Can you work these out from the model? Positions are in its coordinate system, mm. Give positions to 0.01 mm unless a question says otherwise; leave off trailing zeros. Loops run counter-clockwise (first coordinate to the right, second up) from the corner with the lowest first, then second, coordinate; pieces in that order, holes last. Notation, with made-up numbers: (72.25, 72) -> (91.25, 72) arc R24 ccw to (91.25, 102) -> close; hole circle Ø1 at (65, -29). An arc over 180 degrees is marked (long way). Return JSON: item names as keys, results as strings. Group by question number.
Q1. Suppose I cut it at B-B, the plane x = 0. Please give me the cut outline in (y, z), and give its area (3 significant figures).
Q2. Suppose I cut it at C-C, the plane z = 1.3. Please give me the cut outline in (x, y).
Q3. Suppose I cut it at A-A, the plane y = 0. Please give me the cut outline in (x, z), and give its area (3 significant figures).
Q4. I need wall thicknesses on line 1 along X through (y, z) = (2, 0.7); line 2 along X through (y, z) = (25.5, 2.9); line 3 along Y through (x, z) = (29, 0.85). Which ranges of each line are inside material? Lowest first, please. Write a range as [from, to].
Q5. Thinking about a two-plate mould opening in Y: for faces 1 (the flat face through (18, 1, 3)), 2 (the cylindrical face through (24, 0, 1)), 3 (the cylindrical face through (-15.584, 20.234, 1.479)), 4 (the cylindrical face through (-64.49, 59.14, 1.48)), which applies, pulls with the +Y half, pulls with the -Y half, needs draft (parallel to the pull), parting line crosses it, or undercut?
Q6. Suppose I cut it at D-D, the plane x = 29. Please give me the cut outline in (y, z), and give its area (3 significant figures).
Q7. Will these pins go through, and if not, where does the flat tip stop? pin 1 (1.5 mm diameter, centred on x = -43, z = 1, fed in from -Y); pin 2 (9 mm diameter, centred on x = -14.5, y = 25.11, fed in from +Z); pin 3 (1.5 mm diameter, centred on x = -52, y = 46.5, fed in from -Z).
```python
from build123d import *

# Parameters (mm, degrees)
SKETCH1_R           = 87.5
SKETCH1_R_2         = 5
SKETCH1_R_3         = 15
BOSS_EXTRUDE1_DEPTH = 3


with BuildPart() as part:
    # Sketch1 → Boss-Extrude1 (new body)
    with BuildSketch(Plane.XY):
        Circle(SKETCH1_R)
        with Locations((29, 0)):
            Circle(SKETCH1_R_2, mode=Mode.SUBTRACT)
        with Locations((-14.5, -25.11473671)):
            Circle(SKETCH1_R_2, mode=Mode.SUBTRACT)
        with Locations((-14.5, 25.11473671)):
            Circle(SKETCH1_R_2, mode=Mode.SUBTRACT)
        Circle(SKETCH1_R_3, mode=Mode.SUBTRACT)
    extrude(amount=BOSS_EXTRUDE1_DEPTH)


solid = part.part
```
Ans:
{
 "1": {"outline": "(-87.5, 0) -> (-15, 0) -> (-15, 3) -> (-87.5, 3) -> close; (15, 0) -> (87.5, 0) -> (87.5, 3) -> (15, 3) -> close", "area": "435 mm^2"},
 "2": {"outline": "circle Ø175 at (0, 0); hole circle Ø10 at (-14.5, -25.11); hole circle Ø10 at (-14.5, 25.11); hole circle Ø30 at (0, 0); hole circle Ø10 at (29, 0)"},
 "3": {"outline": "(-87.5, 0) -> (-15, 0) -> (-15, 3) -> (-87.5, 3) -> close; (15, 0) -> (24, 0) -> (24, 3) -> (15, 3) -> close; (34, 0) -> (87.5, 0) -> (87.5, 3) -> (34, 3) -> close", "area": "405 mm^2"},
 "4": {"line 1": "x = [-87.48, -14.87], [14.87, 24.42], [33.58, 87.48]", "line 2": "x = [-83.7, -19.49], [-9.51, 83.7]", "line 3": "y = [-82.55, -5], [5, 82.55]"},
 "5": {"face 1": "needs draft", "face 2": "undercut", "face 3": "undercut", "face 4": "parting line crosses it"},
 "6": {"outline": "(-82.55, 0) -> (-5, 0) -> (-5, 3) -> (-82.55, 3) -> close; (5, 0) -> (82.55, 0) -> (82.55, 3) -> (5, 3) -> close", "area": "465 mm^2"},
 "7": {"pin 1": "stops at y = -76.62", "pin 2": "passes through", "pin 3": "stops at z = 0"}
}
